from build123d import *

# Parameters (mm, degrees)
F0_W      = 127
F0_H      = 127
F1_DEPTH  = 254
F5_W      = 101.6
F5_H      = 152.4
F6_DEPTH  = 127
F8_R      = 31.75
F9_DEPTH  = 254
F11_W     = 101.6
F11_H     = 25.9214961534
F11_H_2   = 7.62
F12_DEPTH = 25.4


with BuildPart() as f1:
    # F0 (on Top) → F1 (new body)
    with BuildSketch(Plane.XY):
        Rectangle(F0_W, F0_H)
    extrude(amount=F1_DEPTH)

    # F2 (on Front) → F3 (revolve, cut)
    with BuildSketch(Plane.XZ):
        Polygon((12.7, 25.4), (12.7, 0), (118.2309914892, 0), (118.2309914892, 76.2), (12.7, 76.2), (12.7, 38.1), (19.05, 38.1), (19.05, 25.4), align=None)
    revolve(axis=Axis((0, 0, 127.3276656866), (0, 0, 1)), mode=Mode.SUBTRACT)

    # F5 (on offset) → F6 (cut, through all)
    with BuildSketch(Plane.XZ.offset(63.5)):
        with Locations((0, 165.1)):
            Rectangle(F5_W, F5_H)
    extrude(amount=-F6_DEPTH, mode=Mode.SUBTRACT)

    # F8 (on offset) → F9 (cut)
    with BuildSketch(Plane.YZ.offset(63.5)):
        Polygon((-67.3566020369, 261.3644381861), (-66.4902816981, 199.4223662228), (-11.4787761731, 261.3644381861), align=None)
        Polygon((11.4787761731, 261.3644381861), (66.4902816981, 199.4223662228), (67.3566020369, 261.3644381861), align=None)
        with Locations((0, 162.56)):
            Circle(F8_R)
    extrude(amount=-F9_DEPTH, mode=Mode.SUBTRACT)

    # F11 (on offset) → F12 (cut)
    with BuildSketch(Plane.XY.offset(254)):
        with Locations((0, 30.9799711404)):
            Rectangle(F11_W, F11_H)
        with Locations((0, -30.9799711404)):
            Rectangle(F11_W, F11_H)
        with Locations((0, 3.81)):
            Rectangle(F11_W, F11_H_2)
        with Locations((0, -3.81)):
            Rectangle(F11_W, F11_H_2)
    extrude(amount=-F12_DEPTH, mode=Mode.SUBTRACT)


solid = f1.part
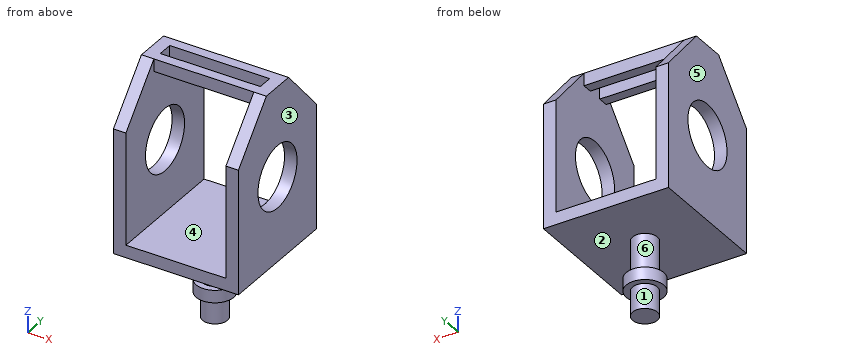
The model under review builds one solid part; all positions refer to its coordinate system, in mm. Face numbers are marked on the shaded views. A direction names the side the tool comes from. Round coordinates to 2 decimals unless told otherwise and drop trailing zeros. Write each loop counter-clockwise with the first axis right and the second up, starting at its lowest first coordinate (ties: lowest second). Pieces come first, ordered by that corner, then holes. Notation, with made-up numbers: (34.5, 22) - (62.5, 22) arc R29 cw to (62.5, 46) - close; hole circle Ø9 at (10, -1.5). An arc over 180 degrees is marked (long way). One line per item, written item: value. Start each with the question number.
1. The part is to be moulded in two halves that separate along X. For the marked faces 1, 2, 3 and 4, say which applies: released by +X, released by -X, zero draft, split by the parting line, or undercut.
2. Consider section C-C on z = 162.56. Write out the cut boundary in (x, y).
3. Consider section D-D on z = 112. Write out the cut boundary in (x, y), and give its area (3 significant figures).
4. Machinability: for the marked faces 5 and 6, which of the approach directions +Z, -Z, +X, -X, +Y, -Y give a long, thin tool a straight path to every point of the face, cutting with its end or side? Answer none if there is none.
5. Consider section B-B on y = 0. Write out the cut boundary in (x, z).
6. Clearance check with flat-ended pins moving along their axes: P1, Ø1, axis at x = 31, y = -16.5, coming from the -Z side; P2, Ø14, axis at x = -14, z = 247, coming from the -Y side; P3, Ø4, axis at x = 24.5, z = 248, coming from the +Y side. State where each tip first meets the part, or that it passes through.
7. To check wall thickness, follow L1, parallel to Z at x = -31, y = 12; L2, parallel to Z at x = 59.75, y = 0; L3, parallel to X at y = 22, z = 189. State the ranges of each line that lie inside material, in increasing order. Write a range as from..to.
8. Consider section A-A on x = -30.5. Write out the cut boundary in (y, z).
Checks:
1. face 1: split by the parting line
1. face 2: zero draft
1. face 3: released by +X
1. face 4: undercut
2. outline: (-63.5, -63.5) - (-50.8, -63.5) - (-50.8, -31.75) - (-63.5, -31.75) - close; (-63.5, 31.75) - (-50.8, 31.75) - (-50.8, 63.5) - (-63.5, 63.5) - close; (50.8, -63.5) - (63.5, -63.5) - (63.5, -31.75) - (50.8, -31.75) - close; (50.8, 31.75) - (63.5, 31.75) - (63.5, 63.5) - (50.8, 63.5) - close
3. outline: (-63.5, -63.5) - (-50.8, -63.5) - (-50.8, 63.5) - (-63.5, 63.5) - close; (50.8, -63.5) - (63.5, -63.5) - (63.5, 63.5) - (50.8, 63.5) - close
3. area: 3,230 mm^2
4. face 5: +Z, -Z, -X, +Y, -Y
4. face 6: none
5. outline: (-63.5, 76.2) - (-12.7, 76.2) - (-12.7, 38.1) - (-19.05, 38.1) - (-19.05, 25.4) - (-12.7, 25.4) - (-12.7, 0) - (12.7, 0) - (12.7, 25.4) - (19.05, 25.4) - (19.05, 38.1) - (12.7, 38.1) - (12.7, 76.2) - (63.5, 76.2) - (63.5, 130.81) - (50.8, 130.81) - (50.8, 88.9) - (-50.8, 88.9) - (-50.8, 130.81) - (-63.5, 130.81) - close; (-63.5, 194.31) - (-50.8, 194.31) - (-50.8, 254) - (-63.5, 254) - close; (50.8, 194.31) - (63.5, 194.31) - (63.5, 254) - (50.8, 254) - close
6. P1: stops at z = 76.2
6. P2: stops at y = -18.02
6. P3: stops at y = 18.02
7. L1: z = 76.2..88.9, 241.3..254
7. L2: z = 76.2..130.81, 194.31..254
7. L3: x = -63.5..-50.8, 50.8..63.5
8. outline: (-63.5, 76.2) - (63.5, 76.2) - (63.5, 88.9) - (-63.5, 88.9) - close; (-18.02, 241.3) - (-7.62, 241.3) - (-7.62, 254) - (-18.02, 254) - close; (7.62, 241.3) - (18.02, 241.3) - (18.02, 254) - (7.62, 254) - close
